Source: CAD feature listing. Evaluate the final solid. Frame: model axes, mm. Face numbers are marked on the shaded views. A direction names the side the tool comes from. Give positions to 0.01 mm unless a question says otherwise; leave off trailing zeros. Order: outer loops, then holes, each group sorted by start corner. A loop starts at its lowest first (then second) coordinate and runs counter-clockwise, first axis right, second up.
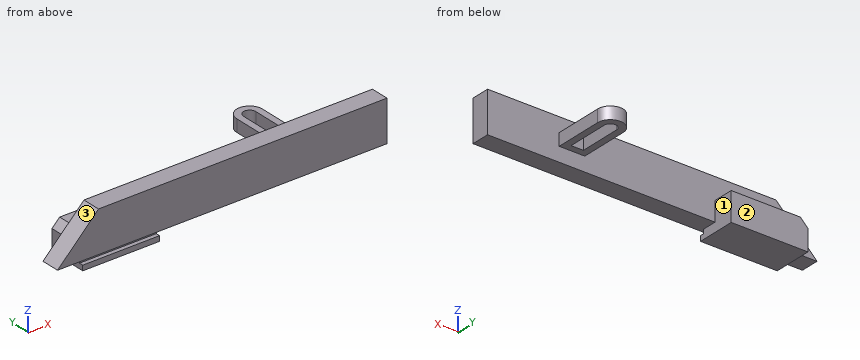
Autodesk Inventor part; units mm, degrees
ref_plane "YZ Plane" through (0, 0, 0) normal (1, 0, 0) x (0, 1, 0)
ref_plane "XZ Plane" through (0, 0, 0) normal (0, 1, 0) x (-1, 0, 0)
ref_plane "XY Plane" through (0, 0, 0) normal (0, 0, 1) x (1, 0, 0)
sketch "Эскиз1" plane through (0, 0, 0) normal (0, 1, 0) x (-1, 0, 0)
  line L0 (-7.5, 2.8) -> (7.5, 2.8)
  line L1 (7.5, 2.8) -> (7.5, -2.8)
  line L2 (7.5, -2.8) -> (-7.5, -2.8)
  line L3 (-7.5, -2.8) -> (-7.5, 2.8)
  line L4 (-7.5, 2.8) -> (7.5, -2.8) construction
  line L5 (7.5, 2.8) -> (-7.5, -2.8) construction
  point P0 (0, 0)
  dimension "d0" = 15
  dimension "d1" = 5.6
extrude "Выдавливание1" add sketch "Эскиз1" along normal blind 7.6
chamfer "Фаска1" distance 1.5 angle 45 1 edges at (-7.5, 3.8, 2.8)
sketch "Эскиз2" plane through (0, 0, 0) normal (0, -1, 0) x (1, 0, 0)
  line L0 (112.65, -2) -> (112.65, 2)
  line L1 (112.65, -2) -> (118.15, -2)
  line L2 (118.15, -2) -> (118.15, -0.4142)
  line L3 (118.15, -0.4142) -> (109.7358, 8)
  line L4 (109.7358, 8) -> (-4.8358, 8)
  line L5 (-4.8358, 8) -> (-13.25, -0.4142)
  line L6 (-13.25, -0.4142) -> (-13.25, -2)
  line L7 (-13.25, -2) -> (-7.75, -2)
  line L8 (-7.75, 2) -> (-7.75, -2)
  line L9 (-6.75, 3) -> (-7.75, 2)
  line L10 (7.75, 3) -> (-6.75, 3)
  line L11 (7.75, -2) -> (7.75, 3)
  line L12 (7.75, -2) -> (97.15, -2)
  line L13 (97.15, 3) -> (97.15, -2)
  line L14 (111.65, 3) -> (97.15, 3)
  line L15 (112.65, 2) -> (111.65, 3)
  line L16 (52.45, 8) -> (52.45, -2) construction
  line L17 (-9.25, -1) -> (-12.4216, -1)
  line L18 (-12.4216, -1) -> (-4.4216, 7)
  line L19 (-4.4216, 7) -> (109.3216, 7)
  line L20 (109.3216, 7) -> (117.3216, -1)
  line L21 (-9.25, -1) -> (117.3216, -1)
  line L22 (52.45, 7) -> (51.95, 7) construction
  line L23 (51.95, 7) -> (51.95, -1)
  line L24 (51.95, -1) -> (52.45, -1) construction
  line L25 (52.45, -1) -> (52.45, 7) construction
  line L26 (72.15, 1.6) -> (66.75, 1.6)
  line L27 (66.75, 1.6) -> (66.75, 4.4)
  line L28 (66.75, 4.4) -> (72.15, 4.4)
  line L29 (72.15, 4.4) -> (72.15, 1.6)
  line L30 (38.15, 1.6) -> (32.75, 1.6)
  line L31 (32.75, 1.6) -> (32.75, 4.4)
  line L32 (32.75, 4.4) -> (38.15, 4.4)
  line L33 (38.15, 4.4) -> (38.15, 1.6)
  point P0 (0, 0)
  point P1 (51.95, 7)
  dimension "d7" = 1
  dimension "d8" = 0.5
extrude "Выдавливание2" add sketch "Эскиз2" against normal blind 3.6 contours L21 L11 L10 L9 L8 L17 L18 L19 L23 | L21 L8 L9 L10 L11 | L30 L31 L32 L33
ref_plane "РабПлоскость1" through (-4.4216, 0, 3) normal (0, 0, 1) x (1, 0, 0)
sketch "Эскиз4" plane through (-4.4216, 0, 3) normal (0, 0, 1) x (1, 0, 0)
  line L0 (56.3716, 0) -> (56.3716, 3.6) construction
  line L1 (56.3716, 3.6) -> (42.3716, 3.6) construction
  line L2 (0, 3.6) -> (56.3716, 3.6) construction
  line L3 (42.3716, 3.6) -> (37.3716, 3.6)
  line L4 (37.3716, 3.6) -> (37.3716, 13.1)
  line L5 (39.8716, 15.6) -> (39.8716, 15.6)
  line L6 (42.3716, 13.1) -> (42.3716, 3.6)
  arc A0 (39.8716, 15.6) -> (37.3716, 13.1) centre (39.8716, 13.1) ccw
  arc A1 (42.3716, 13.1) -> (39.8716, 15.6) centre (39.8716, 13.1) ccw
  line L7 (39.8716, 14.3) -> (39.8716, 14.3)
  arc A2 (39.8716, 14.3) -> (38.6716, 13.1) centre (39.8716, 13.1) ccw
  line L8 (38.6716, 13.1) -> (38.6716, 4.9)
  line L9 (38.6716, 4.9) -> (41.0716, 4.9)
  line L10 (41.0716, 4.9) -> (41.0716, 13.1)
  arc A3 (41.0716, 13.1) -> (39.8716, 14.3) centre (39.8716, 13.1) ccw
  point P0 (4.4216, 0)
  point P1 (37.3716, 15.6)
  point P2 (42.3716, 15.6)
  dimension "d16" = 14
  dimension "d17" = 5
  dimension "d18" = 12
  dimension "d19" = 2.5
  dimension "d20" = 1.3
extrude "Выдавливание3" add sketch "Эскиз4" along normal mid plane 2.4
sketch "Эскиз6" plane through (0, 0, 0) normal (0, -1, 0) x (1, 0, 0)
  line L0 (7.5, -2.8) -> (-7.5, -2.8) construction
  line L1 (7.5, 2.8) -> (7.5, -2.8)
  line L2 (-7.5, -2.8) -> (7.5, -2.8) construction
  line L3 (7.5, -2.8) -> (7.5, -1.8) construction
  line L4 (7.5, -1.8) -> (-7.5, -1.8) construction
  line L5 (-7.5, -1.8) -> (-7.5, -2.8) construction
  line L6 (7.5, -1) -> (51.95, -1)
  line L7 (-7.5, -1.8) -> (7.5, -1.8)
  line L8 (7.5, -1.8) -> (7.5, -1)
  line L9 (7.5, -1) -> (-7.5, -1)
  line L10 (-7.5, -1) -> (-7.5, -1.8)
  point P0 (0, 0)
  dimension "d23" = 1
  dimension "d24" = 15
extrude "Выдавливание4" cut sketch "Эскиз6" against normal blind 0.8
properties part number "microswitch_cap"
1) Section query A-A, the plane y = 6. Return the cut outline in (x, z), and give its area (3 significant figures).
Report:
outline: (-7.5, -2.8) - (7.5, -2.8) - (7.5, 2.8) - (-6, 2.8) - (-7.5, 1.3) - close; (32.95, 1.8) - (34.25, 1.8) - (34.25, 4.2) - (32.95, 4.2) - close; (36.65, 1.8) - (37.95, 1.8) - (37.95, 4.2) - (36.65, 4.2) - close
area: 89.1 mm2
2) Section query B-B, the plane x = 35.45. Return the cut outline in (y, z), and give its area (3 significant figures).
Report:
outline: (0, -1) - (3.6, -1) - (3.6, 1.8) - (4.9, 1.8) - (4.9, 4.2) - (3.6, 4.2) - (3.6, 7) - (0, 7) - close; (14.3, 1.8) - (15.6, 1.8) - (15.6, 4.2) - (14.3, 4.2) - close
area: 35.0 mm2
3) Section query D-D, the plane y = 2.25. Return the cut outline in (x, z).
Report:
outline: (-12.42, -1) - (-7.5, -1) - (-7.5, -2.8) - (7.5, -2.8) - (7.5, -1) - (51.95, -1) - (51.95, 7) - (-4.42, 7) - close
4) Section query C-C, the plane y = 9.75. Return the cut outline in (x, z), and give its area (3 significant figures).
Report:
outline: (32.95, 1.8) - (34.25, 1.8) - (34.25, 4.2) - (32.95, 4.2) - close; (36.65, 1.8) - (37.95, 1.8) - (37.95, 4.2) - (36.65, 4.2) - close
area: 6.24 mm2
5) Material intervals for L1, parallel to X at y = 9.75, z = 3.5; L2, parallel to X at y = 3.75, z = -0.25; L3, parallel to Y at x = 36.5, z = 6.5, sorted ascending.
Report:
L1: x = 32.95 to 34.25, 36.65 to 37.95
L2: x = -7.5 to 7.5
L3: y = 0 to 3.6
6) Reachability of the marked faces 1, 2 and 3 from +Z, -Z, +X, -X, +Y, -Y: full face, straight path, thin tool, end or side. Return the list, or none.
Report:
face 1: -Z, +Y
face 2: +Z, -Z, -X, +Y
face 3: +Z, -X, +Y, -Y
7) Pin query (flat end, axial travel): pin 1 (4 mm diameter, centred on x = 28, y = 1.5, fed in from -Z); pin 2 (1.2 mm diameter, centred on y = 4, z = -1.5, fed in from -X); pin 3 (4 mm diameter, centred on y = 12, z = 0, fed in from -X); pin 4 (3 mm diameter, centred on x = 40.5, y = 10, fed in from -Z). Return the tip coordinate at first contact, or that it passes through.
Report:
pin 1: stops at z = -1
pin 2: stops at x = -7.5
pin 3: stops at x = 32.95
pin 4: passes through
